Build history of the part. All positions in model axes, mm. A direction names the side the tool comes from. Give positions to 0.01 mm unless a question says otherwise; leave off trailing zeros. Loops run counter-clockwise (first coordinate to the right, second up) from the corner with the lowest first, then second, coordinate; pieces in that order, holes last. Notation, with made-up numbers: M 61,30.25 L 72,30.25 A22 ccw 72,44.25 Z; hole C 55,7.25 d7. An arc over 180 degrees is marked long. Put each result on its own line as item: value.
```python
from build123d import *

# Parameters (mm, degrees)
SKETCH1_R           = 2.125
SKETCH1_R_2         = 1.25
SKETCH1_W           = 4.25
SKETCH1_H           = 4.25
BOSS_EXTRUDE1_DEPTH = 20
SKETCH2_W           = 14
SKETCH2_H           = 37
SKETCH2_W_2         = 16
SKETCH2_H_2         = 9
CUT_EXTRUDE1_DEPTH  = 73.470683728
SKETCH3_W           = 33
SKETCH3_H           = 22
BOSS_EXTRUDE2_DEPTH = 14
CUT_EXTRUDE2_DEPTH  = 31
SKETCH5_W           = 16
SKETCH5_H           = 10
CUT_EXTRUDE3_DEPTH  = 29
SKETCH7_R           = 4
CUT_EXTRUDE5_DEPTH  = 2
SKETCH8_W           = 24
SKETCH8_H           = 14
SKETCH8_R           = 1.2
SKETCH8_R_2         = 2.25
BOSS_EXTRUDE3_DEPTH = 6
CUT_EXTRUDE6_START  = -8
SKETCH9_R           = 2.25
SKETCH9_R_2         = 1.2
SKETCH9_W           = 13
SKETCH9_H           = 1.5
CUT_EXTRUDE6_DEPTH  = 8
FILLET1_R           = 8


with BuildPart() as part:
    # Sketch1 → Boss-Extrude1 (new body)
    with BuildSketch(Plane.XY):
        Polygon((16, 54), (0, 54), (0, 0), (60, 0), (60, 14), (16, 14), align=None)
        with Locations((5, 20.5)):
            Circle(SKETCH1_R, mode=Mode.SUBTRACT)
        with Locations((13, 48)):
            Circle(SKETCH1_R_2, mode=Mode.SUBTRACT)
        with Locations((3, 48)):
            Circle(SKETCH1_R_2, mode=Mode.SUBTRACT)
        with Locations((8, 48)):
            Rectangle(SKETCH1_W, SKETCH1_H, mode=Mode.SUBTRACT)
    extrude(amount=BOSS_EXTRUDE1_DEPTH)

    # Sketch2 → Cut-Extrude1 (cut, through all)
    with BuildSketch(Plane(origin=(16, 0, 0), x_dir=(0, 0, -1), z_dir=(1, 0, 0))):
        with Locations((-10, 20.5)):
            Rectangle(SKETCH2_W, SKETCH2_H)
        with Locations((-12, 49.5)):
            Rectangle(SKETCH2_W_2, SKETCH2_H_2)
    extrude(amount=-CUT_EXTRUDE1_DEPTH, mode=Mode.SUBTRACT)

    # Sketch3 → Boss-Extrude2 (add)
    with BuildSketch(Plane.XZ):
        with Locations((43.5, 31)):
            Rectangle(SKETCH3_W, SKETCH3_H)
        with Locations((43.5, -11)):
            Rectangle(SKETCH3_W, SKETCH3_H)
    extrude(amount=-BOSS_EXTRUDE2_DEPTH)

    # Sketch4 → Cut-Extrude2 (cut)
    with BuildSketch(Plane(origin=(60, 0, 0), x_dir=(0, 0, -1), z_dir=(1, 0, 0))):
        Polygon((-18, 0), (-18, 2), (-40, 2), (-40, 12), (20, 12), (20, 2), (-2, 2), (-2, 0), align=None)
    extrude(amount=-CUT_EXTRUDE2_DEPTH, mode=Mode.SUBTRACT)

    # Sketch5 → Cut-Extrude3 (cut)
    with BuildSketch(Plane(origin=(29, 0, 0), x_dir=(0, 0, -1), z_dir=(1, 0, 0))):
        with Locations((-10, 7)):
            Rectangle(SKETCH5_W, SKETCH5_H)
    extrude(amount=-CUT_EXTRUDE3_DEPTH, mode=Mode.SUBTRACT)

    # Sketch7 → Cut-Extrude5 (cut)
    with BuildSketch(Plane.XY.offset(-20)):
        with Locations((45, 7.3)):
            Circle(SKETCH7_R)
    extrude(amount=-CUT_EXTRUDE5_DEPTH, mode=Mode.SUBTRACT)

    # Sketch8 → Boss-Extrude3 (add)
    with BuildSketch(Plane.XY.offset(42)):
        with Locations((48, 7)):
            Rectangle(SKETCH8_W, SKETCH8_H)
        with Locations((57, 7)):
            Circle(SKETCH8_R, mode=Mode.SUBTRACT)
        with Locations((48.25, 7)):
            Circle(SKETCH8_R_2, mode=Mode.SUBTRACT)
        with Locations(Location((39.5, 7, 0), (0, 0, 180))):
            Circle(SKETCH8_R, mode=Mode.SUBTRACT)
    extrude(amount=BOSS_EXTRUDE3_DEPTH)

    # Sketch9 → Cut-Extrude6 (cut)
    with BuildSketch(Plane.XY.offset(48).offset(CUT_EXTRUDE6_START)):
        with Locations((48.25, 7)):
            Circle(SKETCH9_R)
        with Locations((57, 7)):
            Circle(SKETCH9_R_2)
        with Locations(Location((39.5, 7, 0), (0, 0, 180))):
            Circle(SKETCH9_R_2)
        with Locations((53.5, 2.75)):
            Rectangle(SKETCH9_W, SKETCH9_H)
    extrude(amount=CUT_EXTRUDE6_DEPTH, mode=Mode.SUBTRACT)

    # Fillet1
    # the kernel refuses this fillet: 8 mm, written as the material it adds along each edge
    with BuildSketch(Plane(origin=(16, 14, 0), x_dir=(0, 1, 0), z_dir=(0, 0, 1)), Plane(origin=(16, 14, 17), x_dir=(0, 1, 0), z_dir=(0, 0, 1))) as fillet1_piece_1:
        with BuildLine():
            CenterArc((FILLET1_R, -FILLET1_R), FILLET1_R, 90, 90)
            Line((0, -FILLET1_R), (0, 0))
            Line((0, 0), (FILLET1_R, 0))
        make_face()
    extrude(amount=3)
    with BuildSketch(Plane(origin=(16, 14, -20), x_dir=(0, 1, 0), z_dir=(0, 0, 1))) as fillet1_piece_2_section:
        with BuildLine():
            CenterArc((FILLET1_R, -FILLET1_R), FILLET1_R, 90, 90)
            Line((0, -FILLET1_R), (0, 0))
            Line((0, 0), (FILLET1_R, 0))
        make_face()
    fillet1_piece_2 = extrude(amount=43, mode=Mode.PRIVATE)
    fillet1_piece_2 = split(fillet1_piece_2, bisect_by=Plane(origin=(17.786943512, 15.786943512, 17), z_dir=(0, 0, 1)), keep=Keep.TOP, mode=Mode.PRIVATE)
    fillet1_piece_2 = split(fillet1_piece_2, bisect_by=Plane(origin=(17.786943512, 15.786943512, 20), z_dir=(0, 0, -1)), keep=Keep.TOP, mode=Mode.PRIVATE)
    add(fillet1_piece_2)
    with BuildSketch(Plane(origin=(16, 14, -3), x_dir=(0, 1, 0), z_dir=(0, 0, 1))) as fillet1_piece_3_section:
        with BuildLine():
            CenterArc((FILLET1_R, -FILLET1_R), FILLET1_R, 90, 90)
            Line((0, -FILLET1_R), (0, 0))
            Line((0, 0), (FILLET1_R, 0))
        make_face()
    fillet1_piece_3 = extrude(amount=43, mode=Mode.PRIVATE)
    fillet1_piece_3 = split(fillet1_piece_3, bisect_by=Plane(origin=(17.786943512, 15.786943512, 3), z_dir=(0, 0, -1)), keep=Keep.TOP, mode=Mode.PRIVATE)
    fillet1_piece_3 = split(fillet1_piece_3, bisect_by=Plane(origin=(17.786943512, 15.786943512, 0), z_dir=(0, 0, 1)), keep=Keep.TOP, mode=Mode.PRIVATE)
    add(fillet1_piece_3)
    with BuildSketch(Plane(origin=(16, 45, 4), x_dir=(0, 0, 1), z_dir=(-1, 0, 0))) as fillet1_piece_4_section:
        with BuildLine():
            CenterArc((FILLET1_R, FILLET1_R), FILLET1_R, 180, 90)
            Line((0, FILLET1_R), (0, 0))
            Line((0, 0), (FILLET1_R, 0))
        make_face()
    fillet1_piece_4 = extrude(amount=36, mode=Mode.PRIVATE)
    fillet1_piece_4 = fillet1_piece_4 - Plane(origin=(13, 48, 6.838985296), x_dir=(1, 0, 0), z_dir=(0, 0, -1)) * Cylinder(1.25, 105, mode=Mode.PRIVATE)
    fillet1_piece_4 = split(fillet1_piece_4, bisect_by=Plane(origin=(10.125, 45.39955256, 6.838985296), z_dir=(1, 0, 0)), keep=Keep.TOP, mode=Mode.PRIVATE)
    add(fillet1_piece_4)
    with BuildSketch(Plane(origin=(36, 45, 4), x_dir=(0, 0, 1), z_dir=(-1, 0, 0))) as fillet1_piece_5_section:
        with BuildLine():
            CenterArc((FILLET1_R, FILLET1_R), FILLET1_R, 180, 90)
            Line((0, FILLET1_R), (0, 0))
            Line((0, 0), (FILLET1_R, 0))
        make_face()
    fillet1_piece_5 = extrude(amount=36, mode=Mode.PRIVATE)
    fillet1_piece_5 = split(fillet1_piece_5, bisect_by=Plane(origin=(8, 45.875, 6.838985296), z_dir=(0, -1, 0)), keep=Keep.TOP, mode=Mode.PRIVATE)
    fillet1_piece_5 = split(fillet1_piece_5, bisect_by=Plane(origin=(10.125, 45.39955256, 6.838985296), z_dir=(-1, 0, 0)), keep=Keep.TOP, mode=Mode.PRIVATE)
    add(fillet1_piece_5)
    with BuildSketch(Plane(origin=(36, 45, 4), x_dir=(0, 0, 1), z_dir=(-1, 0, 0))) as fillet1_piece_6_section:
        with BuildLine():
            CenterArc((FILLET1_R, FILLET1_R), FILLET1_R, 180, 90)
            Line((0, FILLET1_R), (0, 0))
            Line((0, 0), (FILLET1_R, 0))
        make_face()
    fillet1_piece_6 = extrude(amount=36, mode=Mode.PRIVATE)
    fillet1_piece_6 = split(fillet1_piece_6, bisect_by=Plane(origin=(8, 50.125, 4.159374376), z_dir=(0, 1, 0)), keep=Keep.TOP, mode=Mode.PRIVATE)
    fillet1_piece_6 = split(fillet1_piece_6, bisect_by=Plane(origin=(10.125, 50.838860547, 4.159374376), z_dir=(-1, 0, 0)), keep=Keep.TOP, mode=Mode.PRIVATE)
    add(fillet1_piece_6)
    with BuildSketch(Plane(origin=(36, 45, 4), x_dir=(0, 0, 1), z_dir=(-1, 0, 0))) as fillet1_piece_7_section:
        with BuildLine():
            CenterArc((FILLET1_R, FILLET1_R), FILLET1_R, 180, 90)
            Line((0, FILLET1_R), (0, 0))
            Line((0, 0), (FILLET1_R, 0))
        make_face()
    fillet1_piece_7 = extrude(amount=36, mode=Mode.PRIVATE)
    fillet1_piece_7 = split(fillet1_piece_7, bisect_by=Plane(origin=(5.875, 46.341604388, 7.503816855), z_dir=(-1, 0, 0)), keep=Keep.TOP, mode=Mode.PRIVATE)
    fillet1_piece_7 = fillet1_piece_7 - Plane(origin=(3, 48, 7.503816855), x_dir=(1, 0, 0), z_dir=(0, 0, -1)) * Cylinder(1.25, 105, mode=Mode.PRIVATE)
    add(fillet1_piece_7)
    # the kernel refuses this fillet: 8 mm, written as the material it takes off along each edge
    with BuildSketch(Plane(origin=(0, 0, -20), x_dir=(0, 1, 0), z_dir=(0, 0, 1))) as fillet1_2_piece_1:
        with BuildLine():
            CenterArc((FILLET1_R, -FILLET1_R), FILLET1_R, 90, 90)
            Line((0, -FILLET1_R), (0, 0))
            Line((0, 0), (FILLET1_R, 0))
        make_face()
    extrude(amount=60, mode=Mode.SUBTRACT)
    with BuildSketch(Plane(origin=(36, 45, 20), x_dir=(0, 0, -1), z_dir=(-1, 0, 0))) as fillet1_2_piece_2:
        with BuildLine():
            CenterArc((FILLET1_R, FILLET1_R), FILLET1_R, 180, 90)
            Line((0, FILLET1_R), (0, 0))
            Line((0, 0), (FILLET1_R, 0))
        make_face()
    extrude(amount=56, mode=Mode.SUBTRACT)


solid = part.part
```
Q1. Slice it at B-B (x = 45). List the corners of the cut face in (y, z).
Here are the results:
outline: M 0,-22 L 3.3,-22 L 3.3,-20 L 2,-20 L 2,2 L 0,2 Z; M 0,18 L 2,18 L 2,40 L 12,40 L 12,-20 L 11.3,-20 L 11.3,-22 L 14,-22 L 14,48 L 0,48 Z
Q2. Slice it at D-D (z = -4.5). List the corners of the cut face in (x, y), and give its area (3 significant figures).
Here are the results:
outline: M 27,0 L 60,0 L 60,2 L 29,2 L 29,12 L 60,12 L 60,14 L 27,14 Z
area: 152 mm²
Q3. Slice it at C-C (y = 48). List the corners of the cut face in (x, z) (3 decimals).
Here are the results:
outline: M 0,0 L 1.75,0 L 1.75,5.755 L 0,5.755 Z; M 4.25,0 L 5.875,0 L 5.875,5.755 L 4.25,5.755 Z; M 10.125,0 L 11.75,0 L 11.75,5.755 L 10.125,5.755 Z; M 14.25,0 L 16,0 L 16,5.755 L 14.25,5.755 Z
Q4. Slice it at A-A (x = 25). List the corners of the cut face in (y, z), and give its area (3 significant figures).
Here are the results:
outline: M 0,0 L 14,0 L 14,20 L 0,20 Z; hole M 2,2 L 12,2 L 12,18 L 2,18 Z
area: 120 mm²
Q5. Tool access for faces 4 (the flat face through (16, 39.3, 7.1)), 5 (the flat face through (29, 1, 10)), 6 (the flat face through (27, 7, 31)): list every direction of +Z, -Z, +X, -X, +Y, -Y with a clear straight run to the whole face (end or side of a thin tool).
Here are the results:
face 4: +Z, -Z, +X, +Y
face 5: +X, -Y
face 6: +Z, -X, +Y, -Y
Q6. Probe line 1 (X direction, y = 48, z = 5) (3 decimals); line 2 (Y direction, x = 13, z = 3.15); line 3 (Y direction, x = 53, z = 31.5). List the from-to ranges inside material, lowest first. Write a range as from..to.
Here are the results:
line 1: 0..1.75, 4.25..5.875, 10.125..11.75, 14.25..16
line 2: 0..2, 39..46.75, 49.25..54
line 3: 0..2, 12..14
Q7. Drop flat-ended pins along their axis: pin 1 Ø4 at (x, y) = (13, 48) entering from -Z; pin 2 Ø3 at (x, y) = (3, 48) entering from +Z; pin 3 Ø6 at (y, z) = (28.5, 16.5) entering from +X. Give the stop position or say it passes through.
Here are the results:
pin 1: z = 0
pin 2: z = 7.34
pin 3: x = 16
Q8. Mould opens along X. For faces 1 (the cylindrical face through (3.31, 19.21, 18.48)), 2 (the cylindrical face through (4.54, 0.787, 9.86)), 3 (the flat face through (45, 1, 18)) say: pulls with the +X half, pulls with the -X half, needs draft (parallel to the pull), parting line crosses it, or undercut.
Here are the results:
face 1: undercut
face 2: pulls with the -X half
face 3: needs draft
